from build123d import *

# Parameters (mm, degrees)
SKETCH1_W           = 176
SKETCH1_H           = 84.5
BOSS_EXTRUDE1_DEPTH = 3
SKETCH2_W           = 8
SKETCH2_H           = 5
BOSS_EXTRUDE2_DEPTH = 3
SKETCH3_R           = 1.5
CUT_EXTRUDE1_DEPTH  = 3
SKETCH4_W           = 3
SKETCH4_H           = 8
BOSS_EXTRUDE3_DEPTH = 74.5
CUT_EXTRUDE2_DEPTH  = 3.1
FILLET3_R           = 2.5
FILLET4_R           = 2.5
FILLET7_R           = 2.5
LPATTERN1_COUNT     = 3
LPATTERN1_PITCH     = 25


with BuildPart() as part:
    # Sketch1 → Boss-Extrude1 (new body)
    with BuildSketch(Plane.XY):
        with Locations((88, -42.25)):
            Rectangle(SKETCH1_W, SKETCH1_H)
    extrude(amount=BOSS_EXTRUDE1_DEPTH)

    # Sketch2 → Boss-Extrude2 (add)
    with BuildSketch(Plane(origin=(176, 0, 0), x_dir=(0, 0, -1), z_dir=(1, 0, 0))):
        with Locations((1, -2.5)):
            Rectangle(SKETCH2_W, SKETCH2_H)
    boss_extrude2 = extrude(amount=BOSS_EXTRUDE2_DEPTH)

    # Sketch3 → Cut-Extrude1 (cut)
    with BuildSketch(Plane.ZY.offset(-176)):
        with Locations((-2.5, -2.5)):
            Circle(SKETCH3_R)
    cut_extrude1 = extrude(amount=-CUT_EXTRUDE1_DEPTH, mode=Mode.SUBTRACT)

    # Mirror3: Boss-Extrude2, Cut-Extrude1 across plane
    add(boss_extrude2.mirror(Plane(origin=(0, -42.25, 0), x_dir=(0, 0, 1), z_dir=(0, -1, 0))))
    add(cut_extrude1.mirror(Plane(origin=(0, -42.25, 0), x_dir=(0, 0, 1), z_dir=(0, -1, 0))), mode=Mode.SUBTRACT)

    # Sketch4 → Boss-Extrude3 (add)
    with BuildSketch(Plane(origin=(0, -79.5, 0), x_dir=(1, 0, 0), z_dir=(0, 1, 0))):
        with Locations((177.5, 1)):
            Rectangle(SKETCH4_W, SKETCH4_H)
    extrude(amount=BOSS_EXTRUDE3_DEPTH)

    # Sketch12 → Cut-Extrude2 (cut)
    with BuildSketch(Plane(origin=(0, -70, 0), x_dir=(-1, 0, 0), z_dir=(0, -1, 0))):
        with BuildLine():
            Line((-176, -2.5), (-176, 0))
            Line((-176, 0), (-176, 5))
            Line((-176, 5), (-178.5, 5))
            Line((-178.5, 5), (-178.5, 0))
            ThreePointArc((-178.5, 0), (-177.767766953, -1.767766953), (-176, -2.5))
        make_face()
    cut_extrude2 = extrude(amount=-CUT_EXTRUDE2_DEPTH, mode=Mode.SUBTRACT)

    # Fillet3
    fillet3_edges = [part.edges().sort_by_distance(p)[0] for p in [
        (179, -42.25, 3),
    ]]
    fillet(fillet3_edges, radius=FILLET3_R)

    # Fillet4
    # the kernel refuses this fillet: 2.5 mm, written as the material it takes off along each edge
    with BuildSketch(Plane(origin=(179, -84.5, 0.5), x_dir=(0, 1, 0), z_dir=(0, 0, -1))) as fillet4_piece_1:
        with BuildLine():
            CenterArc((FILLET4_R, -FILLET4_R), FILLET4_R, 90, 90)
            Line((0, -FILLET4_R), (0, 0))
            Line((0, 0), (FILLET4_R, 0))
        make_face()
    extrude(amount=11.75, mode=Mode.SUBTRACT)
    with BuildSketch(Plane(origin=(176.5, -84.5, 0.5), x_dir=(0, 0, 1), z_dir=(-1, 0, 0))) as fillet4_piece_2:
        with BuildLine():
            CenterArc((2.5 - FILLET4_R, FILLET4_R), FILLET4_R, 270, 90)
            Line((2.5 - FILLET4_R, 0), (2.5, 0))
            Line((2.5, 0), (2.5, FILLET4_R))
        make_face()
    revolve(axis=Axis((176.5, -84.5, 0.5), (0, 1, 0)), revolution_arc=90, mode=Mode.SUBTRACT)
    with BuildSketch(Plane(origin=(-6.25, -84.5, 3), x_dir=(0, 1, 0), z_dir=(1, 0, 0))) as fillet4_piece_3:
        with BuildLine():
            CenterArc((FILLET4_R, -FILLET4_R), FILLET4_R, 90, 90)
            Line((0, -FILLET4_R), (0, 0))
            Line((0, 0), (FILLET4_R, 0))
        make_face()
    extrude(amount=182.75, mode=Mode.SUBTRACT)

    # Fillet7
    # the kernel refuses this fillet: 2.5 mm, written as the material it takes off along each edge
    with BuildSketch(Plane(origin=(179, 0, 0.5), x_dir=(-1, 0, 0), z_dir=(0, 0, -1))) as fillet7_piece_1:
        with BuildLine():
            CenterArc((FILLET7_R, -FILLET7_R), FILLET7_R, 90, 90)
            Line((0, -FILLET7_R), (0, 0))
            Line((0, 0), (FILLET7_R, 0))
        make_face()
    extrude(amount=11.75, mode=Mode.SUBTRACT)
    with BuildSketch(Plane(origin=(-6.25, 0, 3), x_dir=(0, 0, -1), z_dir=(1, 0, 0))) as fillet7_piece_2:
        with BuildLine():
            CenterArc((FILLET7_R, -FILLET7_R), FILLET7_R, 90, 90)
            Line((0, -FILLET7_R), (0, 0))
            Line((0, 0), (FILLET7_R, 0))
        make_face()
    extrude(amount=182.75, mode=Mode.SUBTRACT)
    with BuildSketch(Plane(origin=(176.5, 0, 0.5), x_dir=(0, 0, 1), z_dir=(-1, 0, 0))) as fillet7_piece_3:
        with BuildLine():
            CenterArc((2.5 - FILLET7_R, -FILLET7_R), FILLET7_R, 0, 90)
            Line((2.5, -FILLET7_R), (2.5, 0))
            Line((2.5, 0), (2.5 - FILLET7_R, 0))
        make_face()
    revolve(axis=Axis((176.5, 0, 0.5), (0, 1, 0)), revolution_arc=90, mode=Mode.SUBTRACT)

    # LPattern1: Cut-Extrude2 ×3
    with Locations(*[(0, i * LPATTERN1_PITCH, 0) for i in range(1, LPATTERN1_COUNT)]):
        add(cut_extrude2, mode=Mode.SUBTRACT)


solid = part.part
The model under review builds one solid part; all positions refer to its coordinate system, in mm. A direction names the side the tool comes from. Round coordinates to 2 decimals unless told otherwise and drop trailing zeros. Loops run counter-clockwise (first coordinate to the right, second up) from the corner with the lowest first, then second, coordinate; pieces in that order, holes last. Notation, with made-up numbers: M 4.5,-14.5 L 45.5,-14.5 A23 ccw 45.5,1.5 Z; hole C 25,1.25 d1. An arc over 180 degrees is marked long. Answer as a JSON object with one key per item and string values.
Item 1: We need section A-A, the plane z = -2.5. State the section outline as (x, y) points, and give its area (3 significant figures).
Check sheet entries:
{"outline": "M 176,-84.5 L 176.5,-84.5 A2.5 ccw 178.5,-83.5 L 176,-83.5 Z; M 176,-80.5 L 179,-80.5 L 179,-4 L 176,-4 L 176,-16.9 L 178.5,-16.9 L 178.5,-20 L 176,-20 L 176,-41.9 L 178.5,-41.9 L 178.5,-45 L 176,-45 L 176,-66.9 L 178.5,-66.9 L 178.5,-70 L 176,-70 Z; M 176,-1 L 178.5,-1 A2.5 ccw 176.5,0 L 176,0 Z", "area": "210 mm2"}
Item 2: Clearance check with flat-ended pins moving along their axes: P1, Ø4, axis at y = -76.5, z = -3.5, coming from the -X side; P2, Ø0.8, axis at y = -42.5, z = 1.5, coming from the +X side; P3, Ø2, axis at x = 178, z = -2, coming from the -Y side. State where each tip first meets the part, or that it passes through.
Check sheet entries:
{"P1": "x = 176", "P2": "x = 178.93", "P3": "y = -84.45"}
Item 3: For line 1 along Y through (x, z) = (177.5, -2.5); line 2 along Y through (x, z) = (176.7, -2.5); line 3 along X through (y, z) = (-4, -3), list the stretches that pass through material, from the lowest coordinate up.
Check sheet entries:
{"line 1": "-84.29 to -83.5, -80.5 to -70, -66.9 to -45, -41.9 to -20, -16.9 to -4, -1 to -0.21", "line 2": "-84.49 to -83.5, -80.5 to -70, -66.9 to -45, -41.9 to -20, -16.9 to -4, -1 to -0.01", "line 3": "176 to 179"}
Item 4: We need section B-B, the plane y = -31.5. State the section outline as (x, z) points, and give its area (3 significant figures).
Check sheet entries:
{"outline": "M 0,0 L 176,0 L 176,-5 L 179,-5 L 179,0.5 A2.5 ccw 176.5,3 L 0,3 Z", "area": "551 mm2"}
Item 5: The part is to be moulded in two halves that separate along Y. For faces 4 (the face through (87.8, 0, 0.2)), 5 (the face through (176, -31, -2)), 6 (the face through (177.48, -80.67, -1.81)), say which applies: +Y half, -Y half, draft (parallel to the pull), parting line (faces both ways), or undercut.
Check sheet entries:
{"face 4": "+Y half", "face 5": "draft", "face 6": "undercut"}
Item 6: Tool access review of faces 1 (the face through (178.5, -68, -3)), 2 (the face through (176, -56, -2)), 3 (the face through (178.8, -42.8, -5)): name each direction out of +Z, -Z, +X, -X, +Y, -Y from which nothing blocks a thin tool from reaching the whole face with its end or side.
Check sheet entries:
{"face 1": "-Z, -X", "face 2": "-Z, -X, +Y, -Y", "face 3": "-Z, +X, -X, +Y, -Y"}
Item 7: We need section C-C, the plane x = 32. State the section outline as (y, z) points.
Check sheet entries:
{"outline": "M -84.5,0 L 0,0 L 0,0.5 A2.5 ccw -2.5,3 L -82,3 A2.5 ccw -84.5,0.5 Z"}
